Work out the finished part from the listing and answer in its coordinate system (mm). Give positions to 0.01 mm unless a question says otherwise; leave off trailing zeros. Loops run counter-clockwise (first coordinate to the right, second up) from the corner with the lowest first, then second, coordinate; pieces in that order, holes last. Notation, with made-up numbers: (-26.75, 87.25) - (20.25, 87.25) arc R12 ccw to (20.25, 96.25) - close; hole circle Ø9 at (-11, 75.25). An arc over 180 degrees is marked (long way). One line per item, written item: value.
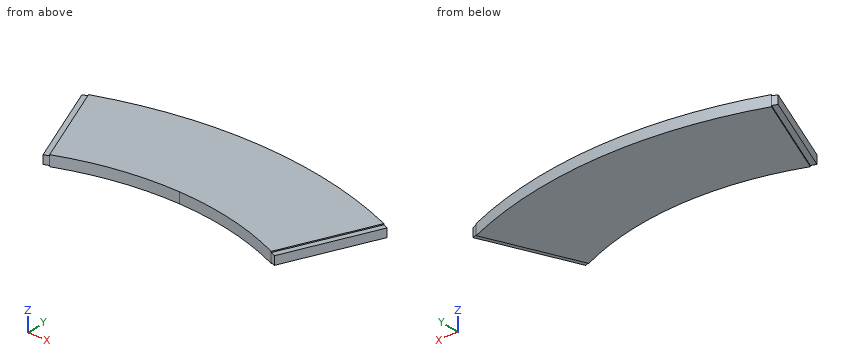
from build123d import *

# Parameters (mm, degrees)
F1_DEPTH = 10
F2_W     = 89.8676701995
F2_H     = 8
F3_DEPTH = 5
F4_W     = 89.8676701995
F4_H     = 8
F5_DEPTH = 5


# Not quite as in the source:
# - a feature names something its author has since deleted; it is built from what else it names


with BuildPart() as f1:
    # F0 (on Top) → F1 (new body)
    with BuildSketch(Plane.XY):
        with BuildLine():
            Line((0, 0), (-140, 0))
            Line((-140, 0), (-105, -82.771964741))
            ThreePointArc((-105, -82.771964741), (-53.5397048927, -67.0734402774), (0, -61.771964741))
            Line((0, -61.771964741), (0, 0))
        make_face()
        with BuildLine():
            Line((140, 0), (0, 0))
            Line((0, 0), (0, -61.771964741))
            ThreePointArc((0, -61.771964741), (53.5397048927, -67.0734402774), (105, -82.771964741))
            Line((105, -82.771964741), (140, 0))
        make_face()
        with BuildLine():
            ThreePointArc((0, 26.228035259), (-71.217817001, 19.6144809107), (-140, 0))
            Line((-140, 0), (0, 0))
            Line((0, 0), (0, 26.228035259))
        make_face()
        with BuildLine():
            Line((0, 26.228035259), (0, 0))
            Line((0, 0), (140, 0))
            ThreePointArc((140, 0), (71.217817001, 19.6144809107), (0, 26.228035259))
        make_face()
    extrude(amount=F1_DEPTH)

    # F2 (on face) → F3 (join)
    with BuildSketch(Plane(origin=(118.7647607356, -50.2194993045, 0), x_dir=(0.3894615263, 0.9210427349, 0), z_dir=(0.9210427349, -0.3894615263, 0))):
        with Locations((9.5907785808, 5)):
            Rectangle(F2_W, F2_H)
    extrude(amount=F3_DEPTH)

    # F4 (on face) → F5 (join)
    with BuildSketch(Plane(origin=(-118.7647607356, -50.2194993045, 0), x_dir=(0.3894615263, -0.9210427349, 0), z_dir=(-0.9210427349, -0.3894615263, 0))):
        with Locations((-9.5907785808, 5)):
            Rectangle(F4_W, F4_H)
    extrude(amount=F5_DEPTH)


solid = f1.part
1. Section C-C (y = -39) is taken. Write down the section's boundary in (x, z).
Output:
outline: (-128.94, 1) - (-123.51, 1) - (-123.51, 0) - (123.51, 0) - (123.51, 1) - (128.94, 1) - (128.94, 9) - (123.51, 9) - (123.51, 10) - (-123.51, 10) - (-123.51, 9) - (-128.94, 9) - close
2. Find the intervals of material crossed by line 1 along X through (y, z) = (-56, 0.75); line 2 along X through (y, z) = (-45, 9.5); line 3 along Y through (x, z) = (-117, 3), in increasing order.
Output:
line 1: x = -116.32 to 116.32
line 2: x = -120.97 to 120.97
line 3: y = -67.23 to 8.11
3. Section B-B (z = 6.25) is taken. Write down the section's boundary in (x, y).
Output:
outline: (-144.61, -1.95) - (-109.61, -84.72) - (-105, -82.77) arc R273 cw to (105, -82.77) - (109.61, -84.72) - (144.61, -1.95) - (140, 0) arc R386.76 ccw to (-140, 0) - close
4. Section A-A (y = -67) is taken. Write down the section's boundary in (x, z).
Output:
outline: (-117.1, 1) - (-111.67, 1) - (-111.67, 0) - (-53.17, 0) - (-53.17, 10) - (-111.67, 10) - (-111.67, 9) - (-117.1, 9) - close; (53.17, 0) - (111.67, 0) - (111.67, 1) - (117.1, 1) - (117.1, 9) - (111.67, 9) - (111.67, 10) - (53.17, 10) - close
5. Section D-D (x = -78) is taken. Write down the section's boundary in (y, z), and give its area (3 significant figures).
Output:
outline: (-73.15, 0) - (18.28, 0) - (18.28, 10) - (-73.15, 10) - close
area: 914 mm²
6. Flat-ended cylindrical pins translate along their axes: pin 1 Ø10 at (x, y) = (43, -24.5) entering from -Z; pin 2 Ø6 at (x, y) = (-18, -68) entering from +Z; pin 3 Ø1 at (y, z) = (-1, 9) entering from -X; pin 4 Ø1.5 at (y, z) = (-21, 7) entering from -X. Find the tip coordinate at first contact, or state that the pin passes through.
Output:
pin 1: stops at z = 0
pin 2: passes through
pin 3: stops at x = -143.55
pin 4: stops at x = -136.87
